Study the drawing (mm; zero at the part's minimum x, y, z) and answer. A direction names the side the tool comes from. Round coordinates to 2 decimals unless told otherwise and drop trailing zeros. Loops run counter-clockwise (first coordinate to the right, second up) from the corner with the lowest first, then second, coordinate; pieces in that order, holes last. Notation, with made-up numbers: (17, 28.25) -> (27, 28.25) arc R27 cw to (27, 51.25) -> close; hole circle Ø11 at (32, 53). An arc over 180 degrees is marked (long way). Use one line per item in the form item = value.
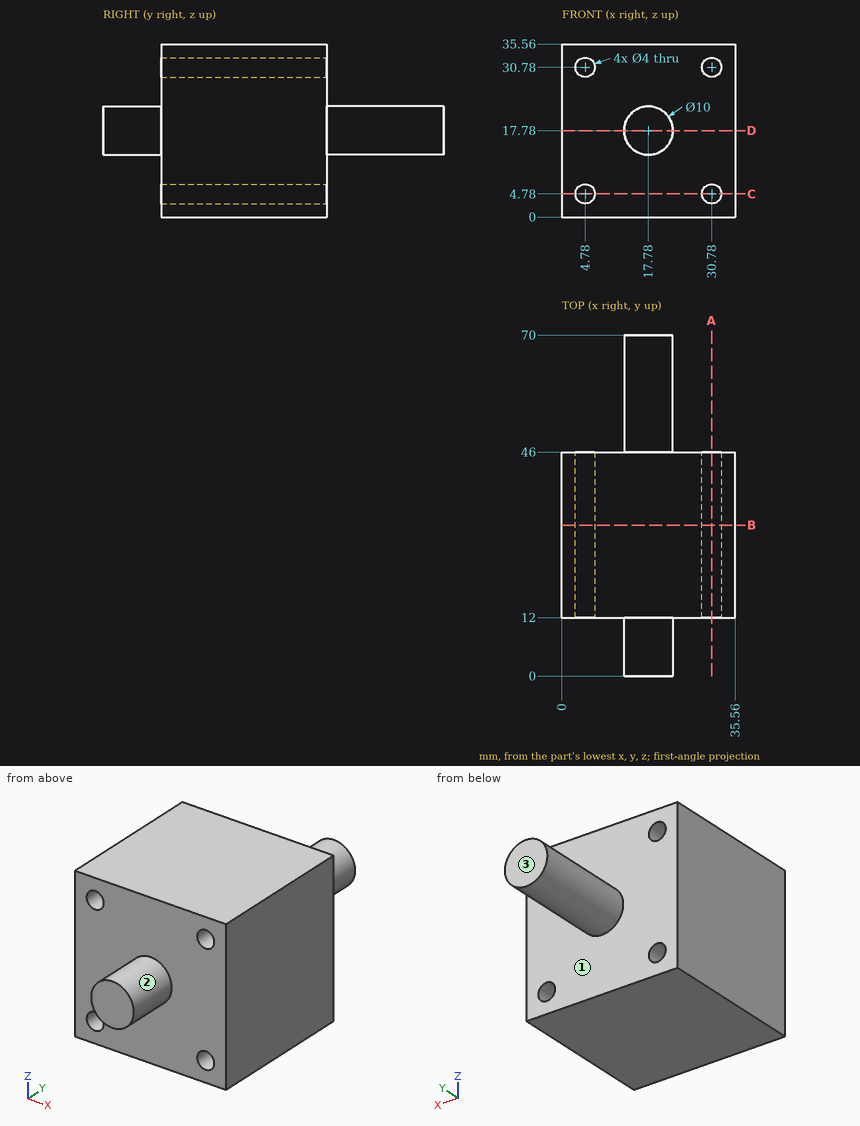
(1) Find section A-A, the plane x = 30.78. Write down the section's boundary in (y, z), then the cut area to 3 significant figures.
Completed:
outline = (12, 0) -> (46, 0) -> (46, 2.78) -> (12, 2.78) -> close; (12, 6.78) -> (46, 6.78) -> (46, 28.78) -> (12, 28.78) -> close; (12, 32.78) -> (46, 32.78) -> (46, 35.56) -> (12, 35.56) -> close
area = 937 mm2
(2) Find section B-B, the plane y = 31. Write down the section's boundary in (x, z), then the cut area to 3 significant figures.
Completed:
outline = (0, 0) -> (35.56, 0) -> (35.56, 35.56) -> (0, 35.56) -> close; hole circle Ø4 at (4.78, 4.78); hole circle Ø4 at (4.78, 30.78); hole circle Ø4 at (30.78, 4.78); hole circle Ø4 at (30.78, 30.78)
area = 1,210 mm2
(3) For the marked faces 1, 2 and 3, determine the directions among +Z, -Z, +X, -X, +Y, -Y from which every point of the face is accessible in a straight line to the end or side of a thin tool.
Completed:
face_1 = +Y
face_2 = -Y
face_3 = +Z, -Z, +X, -X, +Y
(4) Find section C-C, the plane z = 4.78. Write down the section's boundary in (x, y).
Completed:
outline = (0, 12) -> (2.78, 12) -> (2.78, 46) -> (0, 46) -> close; (6.78, 12) -> (28.78, 12) -> (28.78, 46) -> (6.78, 46) -> close; (32.78, 12) -> (35.56, 12) -> (35.56, 46) -> (32.78, 46) -> close
(5) Consider L1, parallel to Z at x = 30.78, y = 38.5; L2, parallel to Z at x = 6, y = 29. Determine where each line is inside the solid, lowest interval first.
Completed:
L1 = 0 to 2.78, 6.78 to 28.78, 32.78 to 35.56
L2 = 0 to 3.2, 6.36 to 29.2, 32.36 to 35.56
(6) Given P1, Ø4, axis at x = 18.5, z = 16.5, coming from the -Y side; P2, Ø1, axis at x = 13.5, y = 52.5, coming from the +Z side; P3, Ø5, axis at x = 24, y = 61, coming from the -Z side; P4, Ø2, axis at y = 47.5, z = 16.5, coming from the +X side, each flat-ended and moving along its own axis, determine where each tip first touches the part or whether it passes through.
Completed:
P1 = 0
P2 = 21.05
P3 = 14.44
P4 = 22.77
(7) Find section D-D, the plane z = 17.78. Write down the section's boundary in (x, y).
Completed:
outline = (0, 12) -> (12.78, 12) -> (12.78, 0) -> (22.78, 0) -> (22.78, 12) -> (35.56, 12) -> (35.56, 46) -> (22.78, 46) -> (22.78, 70) -> (12.78, 70) -> (12.78, 46) -> (0, 46) -> close
